from build123d import *

# Parameters (mm, degrees)
BOSS_EXTRUDE1_DEPTH     = 10
CUT_EXTRUDE1_DEPTH      = 12.489125293
CUT_EXTRUDE1_DEPTH_BACK = 12.489125293
CUT_EXTRUDE2_DEPTH      = 10
SKETCH6_R               = 2.625
CUT_EXTRUDE4_DEPTH      = 1.625
BOSS_EXTRUDE3_REACH     = 14.151
SKETCH7_R               = 2.375
BOSS_EXTRUDE4_START     = -2.375
SKETCH8_R               = 2.375
BOSS_EXTRUDE4_DEPTH     = 2.375
CUT_EXTRUDE6_DEPTH      = 14.416407865
CUT_EXTRUDE6_DEPTH_BACK = 14.416407865
SKETCH11_R              = 1.45
REVOLVE1_ANGLE          = 180
FILLET1_R               = 0.5
FILLET2_R               = 0.5
SKETCH13_W              = 1
SKETCH13_H              = 1
CUT_EXTRUDE7_DEPTH      = 16.7480159
SKETCH14_W              = 1
SKETCH14_H              = 1
CUT_EXTRUDE8_DEPTH      = 17.155494533


with BuildPart() as part:
    # Sketch1 → Boss-Extrude1 (new body)
    with BuildSketch(Plane(origin=(0, 0, 0), x_dir=(1, 0, 0), z_dir=(0, 1, 0))):
        Polygon((-1.333333333, -4), (1.333333333, -4), (4, -1.333333333), (4, 1.333333333), (1.333333333, 4), (-1.333333333, 4), (-4, 1.333333333), (-4, -1.333333333), align=None)
    extrude(amount=BOSS_EXTRUDE1_DEPTH)

    # Sketch2 → Cut-Extrude1 (cut, two sides: drawn at the far end of the back side and taken through both)
    with BuildSketch(Plane(origin=(0, 0, 0), x_dir=(0, 0, -1), z_dir=(1, 0, 0)).offset(-CUT_EXTRUDE1_DEPTH_BACK)):
        Polygon((0, 0), (-4, 0), (-4, 4), align=None)
    extrude(amount=CUT_EXTRUDE1_DEPTH + CUT_EXTRUDE1_DEPTH_BACK, mode=Mode.SUBTRACT)

    # Sketch3 → Cut-Extrude2 (cut)
    with BuildSketch(Plane(origin=(0, 0, 0), x_dir=(1, 0, 0), z_dir=(0, 1, 0))):
        Polygon((0, -3), (-0.5, -2.5), (-0.5, -2), (0.5, -2), (0.5, -2.5), align=None)
        Polygon((0.5, 3), (0.5, 2.5), (0, 2), (-0.5, 2.5), (-0.5, 3), align=None)
    extrude(amount=CUT_EXTRUDE2_DEPTH, mode=Mode.SUBTRACT)

    # Sketch6 → Cut-Extrude4 (cut, symmetric)
    with BuildSketch(Plane(origin=(0, 0, 0), x_dir=(0, 0, -1), z_dir=(1, 0, 0))):
        with Locations((0, -0.5)):
            Circle(SKETCH6_R)
    extrude(amount=CUT_EXTRUDE4_DEPTH, both=True, mode=Mode.SUBTRACT)

    # Boss-Extrude3: up to this face of the body (flat: up to its plane)
    boss_extrude3_end = Plane(part.part.faces().sort_by_distance((-4, 5.157088123, -0.030651341))[0])
    # Sketch7 → Boss-Extrude3 (add, up to the picked face)
    with BuildSketch(Plane(origin=(-1.625, 0, 0), x_dir=(0, 0, -1), z_dir=(1, 0, 0)), mode=Mode.PRIVATE) as boss_extrude3_sk1:
        with Locations((0, -0.5)):
            Circle(SKETCH7_R)
    boss_extrude3_tool1 = split(extrude(boss_extrude3_sk1.sketch, amount=-BOSS_EXTRUDE3_REACH, mode=Mode.PRIVATE), bisect_by=boss_extrude3_end, keep=Keep.BOTH, mode=Mode.PRIVATE)
    add(boss_extrude3_tool1.solids().sort_by(Axis((-1.625, -0.5, 0), (-1, 0, 0)))[0])

    # Sketch8 → Boss-Extrude4 (add)
    with BuildSketch(Plane.ZY.offset(-1.625).offset(BOSS_EXTRUDE4_START)):
        with Locations((0, -0.5)):
            Circle(SKETCH8_R)
    extrude(amount=BOSS_EXTRUDE4_DEPTH)

    # Sketch11 → Cut-Extrude6 (cut, two sides: drawn at the far end of the back side and taken through both)
    with BuildSketch(Plane(origin=(4, 0, 0), x_dir=(0, 0, -1), z_dir=(1, 0, 0)).offset(-CUT_EXTRUDE6_DEPTH_BACK)):
        with Locations((0, -0.5)):
            Circle(SKETCH11_R)
    extrude(amount=CUT_EXTRUDE6_DEPTH + CUT_EXTRUDE6_DEPTH_BACK, mode=Mode.SUBTRACT)

    # Sketch12 → Revolve1 (revolve)
    with BuildSketch(Plane(origin=(0, 10, 0), x_dir=(1, 0, 0), z_dir=(0, 1, 0))):
        Polygon((0, 4), (-1.333333333, 4), (-4, 1.333333333), (-4, -1.333333333), (-1.333333333, -4), (0, -4), align=None)
    revolve(axis=Axis((0, 10, 4), (0, 0, -1)), revolution_arc=REVOLVE1_ANGLE)

    # Fillet1
    # the kernel refuses this fillet: 0.5 mm, written as the material it takes off along each edge
    with BuildSketch(Plane(origin=(4, 0.947645783, 1.333333333), x_dir=(-0.7071067811865454, 0, 0.7071067811865497), z_dir=(0, 1, 0))) as fillet1_piece_1_section:
        with BuildLine():
            CenterArc((FILLET1_R * 0.414213562373, -FILLET1_R), FILLET1_R, 90, 45)
            Line((-FILLET1_R * 0.292893218813, -FILLET1_R * 0.292893218813), (0, 0))
            Line((0, 0), (FILLET1_R * 0.414213562373, 0))
        make_face()
    fillet1_piece_1 = extrude(amount=9.052354217, mode=Mode.PRIVATE)
    fillet1_piece_1 = fillet1_piece_1 - Plane(origin=(3.968890647, -0.5, 0), x_dir=(0, 0, 1), z_dir=(1, 0, 0)) * Cylinder(2.375, 19, mode=Mode.PRIVATE)
    add(fillet1_piece_1, mode=Mode.SUBTRACT)
    with BuildSketch(Plane(origin=(-4, 0.947645783, 1.333333333), x_dir=(0, 0, -1), z_dir=(0, 1, 0))) as fillet1_piece_2_section:
        with BuildLine():
            CenterArc((FILLET1_R * 0.414213562373, -FILLET1_R), FILLET1_R, 90, 45)
            Line((-FILLET1_R * 0.292893218813, -FILLET1_R * 0.292893218813), (0, 0))
            Line((0, 0), (FILLET1_R * 0.414213562373, 0))
        make_face()
    fillet1_piece_2 = extrude(amount=9.052354217, mode=Mode.PRIVATE)
    fillet1_piece_2 = fillet1_piece_2 - Plane(origin=(-3.968890645, -0.5, 0), x_dir=(0, 0, -1), z_dir=(1, 0, 0)) * Cylinder(2.375, 19, mode=Mode.PRIVATE)
    add(fillet1_piece_2, mode=Mode.SUBTRACT)
    with BuildSketch(Plane(origin=(0, 10, 1.333333333), x_dir=(-1, 0, 0), z_dir=(0, -1, 0))) as fillet1_piece_3:
        with BuildLine():
            CenterArc((4 - FILLET1_R, FILLET1_R * 0.414213562373), FILLET1_R, 315, 45)
            Line((4 - FILLET1_R * 0.292893218813, -FILLET1_R * 0.292893218813), (4, 0))
            Line((4, 0), (4, FILLET1_R * 0.414213562373))
        make_face()
    revolve(axis=Axis((0, 10, 1.333333333), (0, 0, -1)), revolution_arc=180, mode=Mode.SUBTRACT)

    # Fillet2
    fillet2_edges = [part.edges().sort_by_distance(p)[0] for p in [
        (4, 5.732706368, -1.333333333),
        (-4, 5.732706368, -1.333333333),
        (0, 14, -1.333333333),
    ]]
    fillet(fillet2_edges, radius=FILLET2_R)

    # Sketch13 → Cut-Extrude7 (cut, through all)
    with BuildSketch(Plane.XY.offset(2)):
        with Locations((0, 9.5)):
            Rectangle(SKETCH13_W, SKETCH13_H)
    extrude(amount=CUT_EXTRUDE7_DEPTH, mode=Mode.SUBTRACT)

    # Sketch14 → Cut-Extrude8 (cut, through all)
    with BuildSketch(Plane.XY.offset(-3)):
        with Locations((0, 9.5)):
            Rectangle(SKETCH14_W, SKETCH14_H)
    extrude(amount=-CUT_EXTRUDE8_DEPTH, mode=Mode.SUBTRACT)


solid = part.part
Read the model definition and answer for the solid it produces. Units are mm, in the model's axes. A direction names the side the tool comes from. Round coordinates to 2 decimals unless told otherwise and drop trailing zeros. Order: outer loops, then holes, each group sorted by start corner. A loop starts at its lowest first (then second) coordinate and runs counter-clockwise, first axis right, second up. Notation, with made-up numbers: (-18.75, 64) - (4.25, 64) arc R24 ccw to (4.25, 88) - close; hole circle Ø1 at (43, -34). An arc over 180 degrees is marked (long way). Use one line per item in the form item = value. Start each with the question number.
(1) The part is cut by section C-C (y = 7). Give the vertices of the cut face in (x, z).
(2) Determine the mould class of faces 1 (the face through (0, 0, -3.2)), 2 (the face through (-2.83, -0.44, 1.45)), 3 (the face through (0, 6, -4)) for opening direction Z: +Z half, -Z half, draft (parallel to the pull), parting line (faces both ways), or undercut.
(3) The part is cut by section D-D (z = -1.75). Give the vertices of the cut face in (x, y) (3 decimals), then the cut area to 3 significant figures.
(4) The part is cut by section A-A (z = 0). Give the vertices of the cut face in (x, y) (3 decimals).
(5) For faces 4 (the face through (0, 10, 3)), 5 (the face through (0, 6, 2)), 6 (the face through (2.576, 6.627, 2.758)), 7 (the face through (-0.5, 6, -2.7)), 8 (the face through (2.611, 4.93, -2.722)), determine the directions among +Z, -Z, +X, -X, +Y, -Y from which every point of the face is accessible in a straight line to the end or side of a thin tool.
(6) The part is cut by section B-B (y = -0.5). Give the vertices of the cut face in (x, z) (3 decimals).
(7) Find the intervals of material crossed by line 1 along Z through (x, y) = (-2.55, -0.5) (3 decimals); line 2 along X through (y, z) = (1, 0) (3 decimals); line 3 along Y through (x, z) = (3.3, 0) (3 decimals), in increasing order. Write a range as from..to.
(8) Flat-ended cylindrical pins translate along their axes: pin 1 Ø1 at (y, z) = (11.5, 3) entering from +X; pin 2 Ø1 at (x, y) = (1.5, 12) entering from -Z; pin 3 Ø4 at (y, z) = (0, 0.5) entering from +X; pin 4 Ø1.1 at (x, z) = (0, -3) entering from -Y. Find the tip coordinate at first contact, or state that the pin passes through.
Checked values:
q1.outline = (-4, -1.13) arc R0.5 ccw to (-3.85, -1.48) - (-1.33, -4) - (1.33, -4) - (3.85, -1.48) arc R0.5 ccw to (4, -1.13) - (4, 1.13) arc R0.5 ccw to (3.85, 1.48) - (1.33, 4) - (-1.33, 4) - (-3.85, 1.48) arc R0.5 ccw to (-4, 1.13) - close; hole (-0.5, -3) - (0.5, -3) - (0.5, -2.5) - (0, -2) - (-0.5, -2.5) - close; hole (-0.5, 2) - (0.5, 2) - (0.5, 2.5) - (0, 3) - (-0.5, 2.5) - close
q2.face_1 = draft
q2.face_2 = undercut
q2.face_3 = -Z half
q3.outline = (-4, -2.106) - (-1.625, -2.106) - (-1.625, 1.457) - (1.625, 1.457) - (1.625, -2.106) - (4, -2.106) - (4, 1.106) - (3.583, 1.106) - (3.583, 10) arc R3.583 ccw to (-3.583, 10) - (-3.583, 1.106) - (-4, 1.106) - close
q3.area = 98.0 mm^2
q4.outline = (-4, -2.875) - (-1.625, -2.875) - (-1.625, -1.95) - (-4, -1.95) - close; (-4, 0.95) - (-1.625, 0.95) - (-1.625, 2.125) - (1.625, 2.125) - (1.625, 0.95) - (4, 0.95) - (4, 10) arc R4 ccw to (-4, 10) - close; (1.625, -2.875) - (4, -2.875) - (4, -1.95) - (1.625, -1.95) - close
q5.face_4 = +Z
q5.face_5 = -Y
q5.face_6 = +Z, +X, +Y
q5.face_7 = none
q5.face_8 = -Z, +X, +Y
q6.outline = (-4, -2.375) - (-1.625, -2.375) - (-1.625, -1.45) - (-4, -1.45) - close; (-4, 1.45) - (-1.625, 1.45) - (-1.625, 2.375) - (-4, 2.375) - close; (1.625, -2.375) - (4, -2.375) - (4, -1.45) - (1.625, -1.45) - close; (1.625, 1.45) - (4, 1.45) - (4, 2.375) - (1.625, 2.375) - close
q7.line_1 = -2.375..-1.45, 1.45..2.375
q7.line_2 = -4..-1.625, 1.625..4
q7.line_3 = -2.875..-1.95, 0.95..12.261
q8.pin_1 = 2.47
q8.pin_2 = -3.33
q8.pin_3 = 4
q8.pin_4 = 0
